Geometry: final body of the model. Coordinates: model frame, mm. Face numbers are marked on the shaded views. A direction names the side the tool comes from. Coordinates: 2 decimals unless noted, no trailing zeros. Write each loop counter-clockwise with the first axis right and the second up, starting at its lowest first coordinate (ties: lowest second). Pieces come first, ordered by that corner, then holes. Notation, with made-up numbers: (34.25, -35) - (55.25, -35) arc R25 cw to (55.25, -15) - close; hole circle Ø2 at (11.5, 29.25). An arc over 180 degrees is marked (long way). Put each result on its own line as item: value.
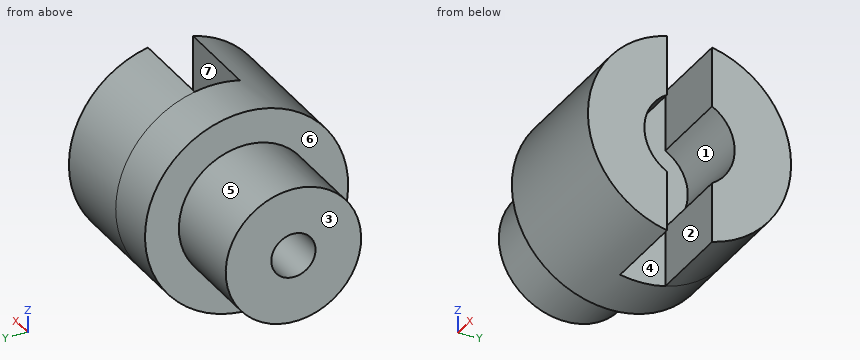
```python
from build123d import *

# Parameters (mm, degrees)
SKETCH_1_R          = 4.5
SKETCH_1_R_2        = 2
EXTRUDE_1_DEPTH     = 4
SKETCH_2_W          = 10.852293239
SKETCH_2_H          = 2
CUT_EXTRUDE_1_DEPTH = 4
SKETCH_5_R          = 4.5
EXTRUDE_3_DEPTH     = 2.5
SKETCH_6_R          = 3
EXTRUDE_4_DEPTH     = 4
SKETCH_7_R          = 0.98
CUT_EXTRUDE_2_DEPTH = 13.278029158


with BuildPart() as part:
    # Sketch 1 → Extrude 1 (new body)
    with BuildSketch(Plane(origin=(0, 0, 0), x_dir=(0, 0, -1), z_dir=(1, 0, 0))):
        Circle(SKETCH_1_R)
        Circle(SKETCH_1_R_2, mode=Mode.SUBTRACT)
    extrude(amount=EXTRUDE_1_DEPTH)

    # Sketch 2 → Cut-Extrude 1 (cut)
    with BuildSketch(Plane(origin=(4, 0, 0), x_dir=(0, 0, -1), z_dir=(1, 0, 0))):
        with Locations((-0.118295573, 0)):
            Rectangle(SKETCH_2_W, SKETCH_2_H)
    extrude(amount=-CUT_EXTRUDE_1_DEPTH, mode=Mode.SUBTRACT)


with BuildPart() as cut_extrude_1_piece_1:
    # of the separate pieces the step leaves, piece 1, a body of its own (cut_extrude_1_pieces)
    add(part.part.solids().sort_by_distance((0, 1, -4.387482194))[0])



with BuildPart() as cut_extrude_1_piece_2:
    # of the separate pieces the step leaves, piece 2, a body of its own (cut_extrude_1_pieces)
    add(part.part.solids().sort_by_distance((0, -1, 4.387482194))[0])


with BuildPart() as cut_extrude_1_piece_1_1:
    add(cut_extrude_1_piece_1.part)

    add(cut_extrude_1_piece_2.part)  # Extrude 3 merges Cut-Extrude 1 piece 2
    # Sketch 5 → Extrude 3 (add)
    with BuildSketch(Plane.ZY):
        Circle(SKETCH_5_R)
    extrude(amount=EXTRUDE_3_DEPTH)

    # Sketch 6 → Extrude 4 (add)
    with BuildSketch(Plane.ZY.offset(2.5)):
        Circle(SKETCH_6_R)
    extrude(amount=EXTRUDE_4_DEPTH)

    # Sketch 7 → Cut-Extrude 2 (cut, through all)
    with BuildSketch(Plane.ZY.offset(6.5)):
        Circle(SKETCH_7_R)
    extrude(amount=-CUT_EXTRUDE_2_DEPTH, mode=Mode.SUBTRACT)


solid = cut_extrude_1_piece_1_1.part
```
1. Set-up query: the marked faces 1, 2 and 3. Return all of +Z, -Z, +X, -X, +Y, -Y with unobstructed straight access to the full face (end or side cutting, diameter ignored); none if empty.
Answer below:
face 1: +X
face 2: +Z, -Z, +X
face 3: +Z, -Z, -X, +Y, -Y
2. Pin query (flat end, axial travel): pin 1 Ø2 at (x, z) = (2.5, -3.5) entering from -Y; pin 2 Ø1.3 at (x, z) = (1, -3) entering from +Y; pin 3 Ø1.8 at (y, z) = (0, 0) entering from +X; pin 4 Ø4 at (x, y) = (-2, -2.5) entering from +Z. Return the tip coordinate at first contact, or that it passes through.
Answer below:
pin 1: stops at y = -3.74
pin 2: stops at y = 3.84
pin 3: passes through
pin 4: stops at z = 4.47
3. Mould query, pull axis Y, two halves, no side actions, for the marked faces 4, 5, 6 and 7. Classes: +Y half, -Y half, draft (parallel to the pull), parting line (faces both ways), or undercut.
Answer below:
face 4: undercut
face 5: parting line
face 6: draft
face 7: undercut
4. Ray query, probe 1 along Y at (x, z) = (3.75, -1); probe 2 along Y at (x, z) = (-3.75, 0); probe 3 along X at (y, z) = (2.25, -2.25). Return the intervals inside material, ascending. Write a range as from..to.
Answer below:
probe 1: y = -4.39..-1.73, 1.73..4.39
probe 2: y = -3..-0.98, 0.98..3
probe 3: x = -2.5..4
5. Section query A-A (x = 2). Return loops of the section in (y, z).
Answer below:
outline: (-1, -4.39) - (-1, -1.73) arc R2 cw to (-1, 1.73) - (-1, 4.39) arc R4.5 ccw to start; (1, -4.39) arc R4.5 ccw to (1, 4.39) - (1, 1.73) arc R2 cw to (1, -1.73) - close
6. Section query B-B (y = 0). Return loops of the section in (x, z).
Answer below:
outline: (-6.5, -3) - (-2.5, -3) - (-2.5, -4.5) - (0, -4.5) - (0, -0.98) - (-6.5, -0.98) - close; (-6.5, 0.98) - (0, 0.98) - (0, 4.5) - (-2.5, 4.5) - (-2.5, 3) - (-6.5, 3) - close
7. Section query D-D (z = -3.25). Return loops of the section in (x, y).
Answer below:
outline: (-2.5, -3.11) - (4, -3.11) - (4, -1) - (0, -1) - (0, 1) - (4, 1) - (4, 3.11) - (-2.5, 3.11) - close
8. Section query C-C (x = -4.75). Return loops of the section in (y, z), then the cut area to 3 significant figures.
Answer below:
outline: circle Ø6 at (0, 0); hole circle Ø1.96 at (0, 0)
area: 25.3 mm²
